Autodesk Fusion 360 part; units mm, degrees
sketch "Skizze1" plane through (0, 0, 0) normal (0, 0, 1) x (1, 0, 0)
  line L0 (-3, 0) -> (-3, 0.8)
  line L1 (-3, 0.8) -> (-2.5, 0.8)
  line L2 (-2.5, 0.8) -> (-2.5, 2.1)
  line L3 (-8.4843, 2.1) -> (11.6981, 2.1) construction
  line L4 (0, 9) -> (0, -6.2163) construction
  arc A0 (0, 4.6) -> (-2.5, 2.1) centre (0, 2.1) ccw
  line L5 (0, 4.6) -> (0, 0)
  line L6 (0, 0) -> (-3, 0)
  line L7 (2.5, 2) -> (4.5, 2)
  line L8 (4.5, 2) -> (4.5, -2)
  line L9 (4.5, -2) -> (2.5, -2)
  line L10 (2.5, -2) -> (2.5, 2)
  line L11 (-2.5, -2) -> (-4.5, -2)
  line L12 (-4.5, -2) -> (-4.5, 2)
  line L13 (-4.5, 2) -> (-2.5, 2)
  line L14 (-2.5, 2) -> (-2.5, -2)
  point P0 (0, 2.1)
  dimension "d1" = 3
  dimension "d2" = 0.8
  dimension "d3" = 2.5
  dimension "d5" = 2.1
  dimension "d7" = 2.5
  dimension "d8" = 2
  dimension "d9" = 2
  dimension "d10" = 2
  dimension "d126" = 2
  dimension "d127" = 2
  dimension "d128" = 2
  dimension "d129" = 2.5
revolve "Drehen1" add sketch "Skizze1" angle 360 about axis through (0, 9, 0) along (0, -1, 0) contours L0 L1 L6 L14 | L2 A0 L5 L6 L14 makes body 1
sketch "Skizze2" plane through (0, 0, 0) normal (0, 0, 1) x (1, 0, 0)
  line L0 (-10, 20) -> (10, 20)
  line L1 (10, 20) -> (10, -6.2)
  line L2 (10, -6.2) -> (-10, -6.2)
  line L3 (-10, -6.2) -> (-10, 20)
  line L4 (0, 21.3723) -> (0, -17) construction
  line L5 (-26.2349, 0) -> (38.3962, 0) construction
  line L6 (5.2, -6.2) -> (5.2, 3.8)
  line L7 (5.2, 3.8) -> (10, 3.8)
  line L8 (-5.2, -6.2) -> (-5.2, 3.8)
  line L9 (-5.2, 3.8) -> (-10, 3.8)
  line L10 (-17, 10) -> (24.4562, 10) construction
  line L11 (-5, 26) -> (-5, 5) construction
  line L12 (5, 25.6741) -> (5, 5) construction
  circle A0 centre (-5, 10) radius 1.75
  circle A1 centre (5, 10) radius 1.75
  line L13 (-16, 15) -> (36.57, 15) construction
  circle A2 centre (0, 15) radius 1.75
  line L14 (-7, 22.2425) -> (-7, -4.6464) construction
  line L15 (7, 22.2425) -> (7, -3.3633) construction
  circle A3 centre (7, 15) radius 1.9
  circle A4 centre (-7, 15) radius 1.9
  dimension "d13" = 10
  dimension "d14" = 10
  dimension "d15" = 6.2
  dimension "d16" = 20
  dimension "d32" = 4.8
  dimension "d33" = 10
  dimension "d34" = 4.8
  dimension "d35" = 10
  dimension "d36" = 10
  dimension "d37" = 5
  dimension "d38" = 5
  dimension "d39" = 3.5
  dimension "d40" = 3.5
  dimension "d41" = 5
  dimension "d42" = 3.5
  dimension "d53" = 7
  dimension "d54" = 7
  dimension "d117" = 3.8
  dimension "d118" = 3.8
extrude "Extrusion2" add sketch "Skizze2" along normal blind 10 separate body contours L0 L1 L2 L3 L6 L7 L8 L9 | L2 L3 L8 L9 | L1 L2 L6 L7 | A0 | A1 | A3 | A4 makes body 2
extrude "Extrusion7" add sketch "Skizze2" against normal blind 3 contours A3 | A4 bodies 2
extrude "Extrusion8" add sketch "Skizze2" against normal blind 9.8 contours L2 L3 L8 L9 | L1 L2 L6 L7 bodies 2
combine "Kombinieren1" operation cut target body 2 tool bodies 1
sketch "Skizze4" plane through (0, 0, 0) normal (0, 0, 1) x (1, 0, 0)
  line L0 (2.15, -6.2) -> (-2.15, -6.2)
  line L1 (-2.15, -6.2) -> (-2.15, 0)
  line L2 (-2.15, 0) -> (2.15, 0)
  line L3 (2.15, 0) -> (2.15, -6.2)
  line L4 (2.15, -6.2) -> (-2.15, 0) construction
  line L5 (-2.15, -6.2) -> (2.15, 0) construction
  line L6 (0, 9.7025) -> (0, -8.7035) construction
  line L7 (-7.2352, -6.2) -> (6.1757, -6.2) construction
  point P0 (0, -3.1)
  point P1 (0, -6.2)
  dimension "d21" = 4.3
  dimension "d22" = 6.2
extrude "Extrusion4" cut sketch "Skizze4" along normal blind 0.25 bodies 2
fillet "Abrundung1" radius 1 1 edges at (-8.7714, 15.6871, -3) on bodies 2
fillet "Abrundung2" radius 1 1 edges at (5.2286, 15.6871, -3) on bodies 2
equation "d3 = Linear Dimension-4"
equation "d5 = 4.6 mm - d"
equation "d7 = Linear Dimension-7"
equation "d129 = Linear Dimension-13"
Model file for the job. Use its own axes, mm. A direction names the side the tool comes from. Coordinates: 2 decimals unless noted, no trailing zeros. Loops run counter-clockwise (first coordinate to the right, second up) from the corner with the lowest first, then second, coordinate; pieces in that order, holes last. Notation, with made-up numbers: (-29, 65.5) - (-24, 65.5) arc R18 cw to (-24, 84.5) - close; hole circle Ø2 at (41, 59.25). An arc over 180 degrees is marked (long way). Answer as a JSON object with one key per item and string values. Group by question number.
(1) Flat gauge pins, fed straight in: pin 1 (0.5 mm diameter, centred on x = 7, y = 15.5, fed in from -Z); pin 2 (4 mm diameter, centred on x = -6.5, z = -6, fed in from +Y); pin 3 (1.3 mm diameter, centred on x = -0.5, y = -4.5, fed in from -Z). Where does each tip first touch, or does it go through?
(2) Cut at C-C (z = 5.75). Give the cut face in (x, y), then the cut area to 3 significant figures.
(3) Tool access for faces 1 (the face through (-5.2, -1, -5)), 2 (the face through (5.6, 16.284, -0.986)), 3 (the face through (-7, 15, -3)), 4 (the face through (8, 3.8, -5)): list every direction of +Z, -Z, +X, -X, +Y, -Y with a clear straight run to the whole face (end or side of a thin tool).
(4) Two-plate mould, pull along Y, no slides. Class faces 5 (the face through (-8, -1, -9.8)), 6 (the face through (-0.228, 13.265, 4.93)), 7 (the face through (0, 20, 5)): released by +Y, released by -Y, zero draft, split by the parting line, or undercut.
(5) Cut at A-A (z = -8.5). Give the cut face in (x, y).
(6) Cut at D-D (y = -1.25). Give the cut face in (x, z).
(7) Cut at B-B (x = 0). Give the cut face in (y, z), then the cut area to 3 significant figures.
(8) Probe line 1 along Y through (x, z) = (0, 8.25); line 2 along Y through (x, z) = (-8.5, -5.75); line 3 along Z through (x, y) = (-2, -0.75). List the from-to ranges inside material, lowest first.
Geometry says:
{
 "1": {"pin 1": "stops at z = -3", "pin 2": "stops at y = 3.8", "pin 3": "stops at z = 0.25"},
 "2": {"outline": "(-10, -6.2) - (10, -6.2) - (10, 20) - (-10, 20) - close; hole circle Ø3.5 at (0, 15)", "area": "514 mm^2"},
 "3": {"face 1": "-Z, -Y", "face 2": "-Z", "face 3": "-Z, +X, -X, +Y", "face 4": "-Z, +X, -X"},
 "4": {"face 5": "zero draft", "face 6": "undercut", "face 7": "released by +Y"},
 "5": {"outline": "(-10, -6.2) - (-5.2, -6.2) - (-5.2, 3.8) - (-10, 3.8) - close; (5.2, -6.2) - (10, -6.2) - (10, 3.8) - (5.2, 3.8) - close"},
 "6": {"outline": "(-10, -9.8) - (-5.2, -9.8) - (-5.2, 0) - (-2.15, 0) - (-2.15, 0.25) - (2.15, 0.25) - (2.15, 0) - (5.2, 0) - (5.2, -9.8) - (10, -9.8) - (10, 10) - (-10, 10) - close"},
 "7": {"outline": "(-6.2, 0.25) - (0, 0.25) - (0, 3) - (0.8, 3) - (0.8, 2.5) - (2.1, 2.5) arc R2.5 cw to (4.6, 0) - (13.25, 0) - (13.25, 10) - (-6.2, 10) - close; (16.75, 0) - (20, 0) - (20, 10) - (16.75, 10) - close", "area": "215 mm^2"},
 "8": {"line 1": "y = -6.2 to 13.25, 16.75 to 20", "line 2": "y = -6.2 to 3.8", "line 3": "z = 0.25 to 10"}
}
